The listing builds one solid part. Answer for the finished solid, in the listing's coordinates (mm). A direction names the side the tool comes from. Round coordinates to 2 decimals unless told otherwise and drop trailing zeros. Loops run counter-clockwise (first coordinate to the right, second up) from the corner with the lowest first, then second, coordinate; pieces in that order, holes last. Notation, with made-up numbers: M -22,22.5 L 29,22.5 A30 cw 29,46.5 Z; hole C 79,-9 d1. An arc over 180 degrees is marked long. Put each result on its own line as item: value. Start each with the question number.
(1) Section D-D, the plane x = 17 is taken. Determine the outline of the cut face in (y, z).
(2) Flat-ended cylindrical pins translate along their axes: P1, Ø1.5, axis at y = 7, z = -8.5, coming from the +X side; P2, Ø1.7, axis at y = 14, z = -3, coming from the +X side; P3, Ø1.8, axis at x = -1, z = -2.5, coming from the +Y side. Find the tip coordinate at first contact, or state that the pin passes through.
(3) Determine the mould class of faces 1 (the face through (8, 0, -5)), 2 (the face through (5.428, 13.384, -19.678)), 3 (the face through (8, 8, -25.4)) for opening direction Z: released by +Z, released by -Z, zero draft, split by the parting line, or undercut.
(4) Section B-B, the plane z = -3.75 is taken. Determine the outline of the cut face in (x, y).
(5) Section C-C, the plane x = 8.15 is taken. Determine the outline of the cut face in (y, z).
(6) Which of the six approach directions +Z, -Z, +X, -X, +Y, -Y give full straight-line access (tool end or side, diameter ignored) to faces 4 (the face through (10, 2, -18.1)), 5 (the face through (4.01, 1.66, -23.32)), 6 (the face through (17, 5.8, -5)), 7 (the face through (17, 10.5, -5))?
(7) Section A-A, the plane y = 8.15 is taken. Determine the outline of the cut face in (x, z), then the cut area to 3 significant figures.
(8) Straight lines are drawn through the part: line 1 (Z direction, x = 14.25, y = 4.25); line 2 (X direction, y = 8, z = -20.75); line 3 (Y direction, x = 16.75, z = -6.75). For each, find the intervals that lie inside material, in ascending order.
Autodesk Inventor part; units mm, degrees
ref_plane "YZ Plane" through (0, 0, 0) normal (1, 0, 0) x (0, 1, 0)
ref_plane "XZ Plane" through (0, 0, 0) normal (0, 1, 0) x (-1, 0, 0)
ref_plane "XY Plane" through (0, 0, 0) normal (0, 0, 1) x (1, 0, 0)
sketch "Эскиз1" plane through (0, 0, 0) normal (0, 0, 1) x (1, 0, 0)
  line L0 (0, 0) -> (16.3, 0)
  line L1 (16.3, 16.3) -> (0, 16.3)
  line L2 (0, 10.5) -> (-1.65, 10.5)
  line L3 (0, 5.8) -> (-1.65, 5.8)
  line L4 (16.3, 10.5) -> (17.95, 10.5)
  line L5 (16.3, 5.8) -> (17.95, 5.8)
  arc A0 (-1.65, 10.5) -> (-1.65, 5.8) centre (-1.65, 8.15) ccw
  arc A1 (17.95, 5.8) -> (17.95, 10.5) centre (17.95, 8.15) ccw
  line L6 (0, 16.3) -> (0, 10.5)
  line L7 (0, 5.8) -> (0, 0)
  line L8 (16.3, 0) -> (16.3, 5.8)
  line L9 (16.3, 10.5) -> (16.3, 16.3)
  point P0 (-4, 8.15)
  dimension "d0" = 4.7
  dimension "d1" = 4
  dimension "d2" = 16.3
  dimension "d3" = 16.3
  dimension "d4" = 4.7
extrude "Выдавливание1" add sketch "Эскиз1" against normal blind 9.5
sketch "Эскиз2" plane through (0, 0, -9.5) normal (0, 0, -1) x (-1, 0, 0)
  circle A0 centre (-8.15, 8.15) radius 7.7
  arc A1 (1.65, 5.8) -> (1.65, 10.5) centre (1.65, 8.15) ccw
  line L0 (0, 16.3) -> (-16.3, 16.3)
  point P0 (0, 0)
  point P1 (4, 8.15)
  point P2 (-8.15, 16.3)
  dimension "d7" = 15.4
extrude "Выдавливание2" add sketch "Эскиз2" along normal blind 8.6
sketch "Эскиз3" plane through (8.15, 8.15, -18.1) normal (0, 0, -1) x (-1, 0, 0)
  circle A0 centre (0, 0) radius 5.9
  dimension "d10" = 11.8
extrude "Выдавливание3" add sketch "Эскиз3" along normal blind 3.2
sketch "Эскиз4" plane through (8.15, 8.15, -21.3) normal (0, 0, -1) x (-1, 0, 0)
  circle A0 centre (0, 0) radius 7.7
extrude "Выдавливание4" add sketch "Эскиз4" along normal blind 4.1
equation "\"d4\" = d0"
properties part number "cum"
Recorded:
1. outline: M 5.8,-9.5 L 10.5,-9.5 L 10.5,0 L 5.8,0 Z
2. P1: stops at x = 20.27
2. P2: stops at x = 16.3
2. P3: stops at y = 10.5
3. face 1: zero draft
3. face 2: undercut
3. face 3: released by -Z
4. outline: M -1.65,5.8 L 0,5.8 L 0,0 L 16.3,0 L 16.3,5.8 L 17.95,5.8 A2.35 ccw 17.95,10.5 L 16.3,10.5 L 16.3,16.3 L 0,16.3 L 0,10.5 L -1.65,10.5 A2.35 ccw Z
5. outline: M 0,-9.5 L 0.45,-9.5 L 0.45,-18.1 L 2.25,-18.1 L 2.25,-21.3 L 0.45,-21.3 L 0.45,-25.4 L 15.85,-25.4 L 15.85,-21.3 L 14.05,-21.3 L 14.05,-18.1 L 15.85,-18.1 L 15.85,-9.5 L 16.3,-9.5 L 16.3,0 L 0,0 Z
6. face 4: none
6. face 5: -Z
6. face 6: +Z, -Z, +X, -Y
6. face 7: +Z, -Z, +X, +Y
7. outline: M -4,-9.5 L 0.45,-9.5 L 0.45,-18.1 L 2.25,-18.1 L 2.25,-21.3 L 0.45,-21.3 L 0.45,-25.4 L 15.85,-25.4 L 15.85,-21.3 L 14.05,-21.3 L 14.05,-18.1 L 15.85,-18.1 L 15.85,-9.5 L 20.3,-9.5 L 20.3,0 L -4,0 Z
7. area: 464 mm²
8. line 1: z = -25.4 to -21.3, -18.1 to 0
8. line 2: x = 2.25 to 14.05
8. line 3: y = 5.8 to 10.5
